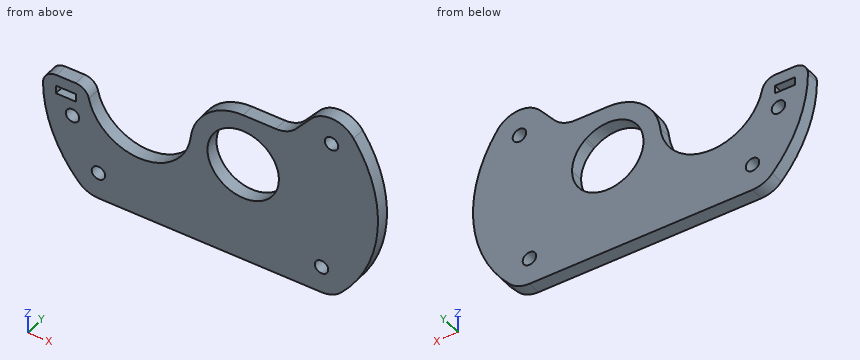
```python
from build123d import *

# Parameters (mm, degrees)
F0_R     = 2.5
F0_W     = 7.5
F0_H     = 3
F1_DEPTH = 5


with BuildPart() as f1:
    # F0 (on Front) → F1 (new body)
    with BuildSketch(Plane.XZ):
        with BuildLine():
            Line((-53.669743, -37.5), (29.047375, -37.5))
            ThreePointArc((29.047375, -37.5), (33.000222, -36.685587), (36.309219, -34.375))
            ThreePointArc((36.309219, -34.375), (49.864682, -3.676068), (40.957602, 28.678822))
            ThreePointArc((40.957602, 28.678822), (33.247823, 32.931447), (25.164572, 29.440522))
            Line((25.164572, 29.440522), (19.7208, 23.071748))
            ThreePointArc((19.7208, 23.071748), (16.304105, 20.486959), (12.11929, 19.569212))
            Line((12.11929, 19.569212), (0, 19.569212))
            ThreePointArc((0, 19.569212), (-13.044872, 14.587166), (-19.447661, 2.177743))
            ThreePointArc((-19.447661, 2.177743), (-37.550938, -14.819453), (-57.215631, 0.344095))
            ThreePointArc((-57.215631, 0.344095), (-58.958953, 3.193251), (-62.107302, 4.308938))
            Line((-62.107302, 4.308938), (-69.242118, 4.308938))
            ThreePointArc((-69.242118, 4.308938), (-72.788821, 2.833268), (-74.242018, -0.722701))
            ThreePointArc((-74.242018, -0.722701), (-70.76408, -18.73091), (-61.026424, -34.273422))
            ThreePointArc((-61.026424, -34.273422), (-57.68632, -36.657899), (-53.669743, -37.5))
        make_face()
        with Locations((-53.669743, -27.5)):
            Circle(F0_R, mode=Mode.SUBTRACT)
        with Locations((-63.29486, -9.063897)):
            Circle(F0_R, mode=Mode.SUBTRACT)
        with Locations((29.047375, -27.5)):
            Circle(F0_R, mode=Mode.SUBTRACT)
        with Locations((-65.67471, -1.5)):
            Rectangle(F0_W, F0_H, mode=Mode.SUBTRACT)
        with BuildLine():
            ThreePointArc((8.60914, 10.072001), (12.033985, 5.54488), (13.25, 0))
            ThreePointArc((13.25, 0), (-11.883564, -5.860325), (8.066089, 10.511932))
            ThreePointArc((8.066089, 10.511932), (8.340516, 10.295547), (8.60914, 10.072001))
        make_face(mode=Mode.SUBTRACT)
        with Locations((32.766082, 22.943057)):
            Circle(F0_R, mode=Mode.SUBTRACT)
    extrude(amount=F1_DEPTH)


solid = f1.part
```
Here's how the part is built. I have some questions about the finished solid (model axes, mm). Give positions to 0.01 mm unless a question says otherwise; leave off trailing zeros. Loops run counter-clockwise (first coordinate to the right, second up) from the corner with the lowest first, then second, coordinate; pieces in that order, holes last. Notation, with made-up numbers: M -31.5,6 L -4.5,6 A28 cw -4.5,44 Z; hole C -12.5,86.25 d6. An arc over 180 degrees is marked long. Return JSON: item names as keys, results as strings.
Item 1: Imagine slicing it at B-B on x = -7.5. List the corners of the cut face in (y, z) for me, then the cut area to 3 significant figures.
A:
{"outline": "M -5,-37.5 L 0,-37.5 L 0,-10.92 L -5,-10.92 Z; M -5,10.92 L 0,10.92 L 0,18.07 L -5,18.07 Z", "area": "169 mm^2"}
Item 2: Please list where these lines run through material, in increasing order: line 1 (X direction, y = -2.7, z = -1); line 2 (X direction, y = -3.1, z = 1); line 3 (X direction, y = -1.2, z = -8).
A:
{"line 1": "x = -74.24 to -69.42, -61.92 to -56.88, -20.08 to -13.21, 13.21 to 49.99", "line 2": "x = -73.95 to -57.4, -19.62 to -13.21, 13.21 to 49.99", "line 3": "x = -73.66 to -65.56, -61.03 to -53.15, -23.81 to -10.56, 10.56 to 49.36"}
Item 3: Imagine slicing it at D-D on z = -17. List the corners of the cut face in (x, y) for me, then the cut area to 3 significant figures.
A:
{"outline": "M -71.41,-5 L 47.02,-5 L 47.02,0 L -71.41,0 Z", "area": "592 mm^2"}
Item 4: I'm going to push flat-ended pins straight in: pin 1 Ø4 at (x, z) = (32.77, 22.94) entering from -Y; pin 2 Ø2.5 at (x, y) = (-64, -3) entering from +Z; pin 3 Ø1.5 at (x, y) = (-66, -1.5) entering from -Z; pin 4 Ø3 at (y, z) = (-4.5, -20) entering from -X. Where does each tip first touch, or does it pass through?
A:
{"pin 1": "passes through", "pin 2": "stops at z = 4.31", "pin 3": "stops at z = -29.01", "pin 4": "stops at x = -70.85"}
Item 5: Imagine slicing it at A-A on z = -27.5. List the corners of the cut face in (x, y) for me.
A:
{"outline": "M -66.27,-5 L -56.17,-5 L -56.17,0 L -66.27,0 Z; M -51.17,-5 L 26.55,-5 L 26.55,0 L -51.17,0 Z; M 31.55,-5 L 41.76,-5 L 41.76,0 L 31.55,0 Z"}
Item 6: Imagine slicing it at C-C on y = -2. List the corners of the cut face in (x, z) for me (3 decimals), then the cut area to 3 significant figures.
A:
{"outline": "M -74.242,-0.723 A50 ccw -61.026,-34.273 A10 ccw -53.67,-37.5 L 29.047,-37.5 A10 ccw 36.309,-34.375 A50 ccw 40.958,28.679 A10 ccw 25.165,29.441 L 19.721,23.072 A10 cw 12.119,19.569 L 0,19.569 A19.569 ccw -19.448,2.178 A19.151 cw -57.216,0.344 A5 ccw -62.107,4.309 L -69.242,4.309 A5 ccw Z; hole M -69.425,-3 L -61.925,-3 L -61.925,0 L -69.425,0 Z; hole C -63.295,-9.064 d5; hole C -53.67,-27.5 d5; hole M 8.066,10.512 A13.25 ccw long 13.25,0 A13.25 ccw 8.609,10.072 A13.251 ccw Z; hole C 29.047,-27.5 d5; hole C 32.766,22.943 d5", "area": "4,790 mm^2"}
